Geometry: final body of the model. Coordinates: model frame, mm. A direction names the side the tool comes from. Coordinates: 2 decimals unless noted, no trailing zeros. Order: outer loops, then holes, each group sorted by start corner. A loop starts at its lowest first (then second) coordinate and runs counter-clockwise, first axis right, second up. Notation, with made-up numbers: (59.5, 3.5) -> (100.5, 3.5) arc R23 cw to (100.5, 25.5) -> close; hole circle Ø11 at (59, -11). An arc over 180 degrees is marked (long way). Answer in a Markdown table with one row per item. Add a question column.
1) Section query C-C on y = -177.8. Return the cut outline in (x, z) (3 decimals), then the cut area to 3 significant figures.
2) Pull-direction query (Y, two-part tool) for faces 3 (the face through (6, 196.85, -1)), 4 (the face through (9.21, -6.64, 124.28)), 5 (the face through (3.131, -46.94, 92.247)); classes: +Y half, -Y half, draft (parallel to the pull), parting line (faces both ways), or undercut.
3) Section query B-B on x = 38. Return the cut outline in (y, z).
4) Section query A-A on z = 44.45. Return the cut outline in (x, y).
5) Section query D-D on y = -93. Return the cut outline in (x, z) (3 decimals), then the cut area to 3 significant figures.
6) Ray query, line 1 (Y direction, x = 4, z = 44); line 2 (Y direction, x = 2.25, z = -44.45); line 3 (Z direction, x = 37.5, y = 130). Return the intervals inside material, ascending. Write a range as from..to.
7) Contact query for a flat-ended pin moving along its axis: P1, Ø1, axis at y = 13.5, z = 49.5, coming from the +X side. Output: stop coordinate, or through.
8) Set-up query: faces 1 (the face through (3.131, -43.793, 52.445)), 2 (the face through (30, -7, 127)). Return all of +Z, -Z, +X, -X, +Y, -Y with unobstructed straight access to the full face (end or side cutting, diameter ignored); none if empty.
```python
from build123d import *

# Parameters (mm, degrees)
BASE_EXTRUDE_THIN_DEPTH      = 196.85
BASE_EXTRUDE_THIN_DEPTH_BACK = 215.9
SKETCH3_R                    = 8.382
HOLES_DEPTH                  = 258.625377244


with BuildPart() as part:
    # Sketch1 → Base-Extrude-Thin (new, two sides)
    with BuildSketch(Plane(origin=(0, 0, 0), x_dir=(1, 0, 0), z_dir=(0, 1, 0))) as base_extrude_thin_sk:
        with BuildLine():
            Line((44.45, 133.35), (15.875, 133.35))
            ThreePointArc((15.875, 133.35), (4.649679849, 128.700320151), (0, 117.475))
            Line((0, 117.475), (0, 0))
            Line((0, 0), (0, -117.475))
            ThreePointArc((0, -117.475), (4.649679849, -128.700320151), (15.875, -133.35))
            Line((15.875, -133.35), (44.45, -133.35))
            Line((44.45, -133.35), (44.45, -127))
            Line((44.45, -127), (15.875, -127))
            ThreePointArc((15.875, -127), (9.139807909, -124.210192091), (6.35, -117.475))
            Line((6.35, -117.475), (6.35, 0))
            Line((6.35, 0), (6.35, 117.475))
            ThreePointArc((6.35, 117.475), (9.139807909, 124.210192091), (15.875, 127))
            Line((15.875, 127), (44.45, 127))
            Line((44.45, 127), (44.45, 133.35))
        make_face()
    extrude(amount=BASE_EXTRUDE_THIN_DEPTH)
    extrude(base_extrude_thin_sk.sketch, amount=-BASE_EXTRUDE_THIN_DEPTH_BACK)

    # Sketch3 (on Right Plane) → holes (cut, through all)
    with BuildSketch(Plane(origin=(0, 0, 0), x_dir=(0, 0, -1), z_dir=(1, 0, 0))):
        with Locations(Location((44.45, 168.275, 0), (0, 0, 180))):
            Circle(SKETCH3_R)
        with Locations(Location((44.45, 41.275, 0), (0, 0, 180))):
            Circle(SKETCH3_R)
        with Locations(Location((44.45, -41.275, 0), (0, 0, 180))):
            Circle(SKETCH3_R)
        with Locations(Location((44.45, -177.8, 0), (0, 0, 180))):
            Circle(SKETCH3_R)
        with Locations(Location((-44.45, -177.8, 0), (0, 0, 180))):
            Circle(SKETCH3_R)
        with Locations(Location((-98.425, -177.8, 0), (0, 0, 180))):
            Circle(SKETCH3_R)
        with Locations(Location((-98.425, -41.275, 0), (0, 0, 180))):
            Circle(SKETCH3_R)
        with Locations(Location((-44.45, -41.275, 0), (0, 0, 180))):
            Circle(SKETCH3_R)
        with Locations(Location((-44.45, 41.275, 0), (0, 0, 180))):
            Circle(SKETCH3_R)
        with Locations(Location((-98.425, 41.275, 0), (0, 0, 180))):
            Circle(SKETCH3_R)
        with Locations(Location((-98.425, 168.275, 0), (0, 0, 180))):
            Circle(SKETCH3_R)
        with Locations(Location((-44.45, 168.275, 0), (0, 0, 180))):
            Circle(SKETCH3_R)
        with Locations(Location((98.425, -177.8, 0), (0, 0, 180))):
            Circle(SKETCH3_R)
        with Locations(Location((98.425, -41.275, 0), (0, 0, 180))):
            Circle(SKETCH3_R)
        with Locations(Location((98.425, 41.275, 0), (0, 0, 180))):
            Circle(SKETCH3_R)
        with Locations(Location((98.425, 168.275, 0), (0, 0, 180))):
            Circle(SKETCH3_R)
    extrude(amount=HOLES_DEPTH, mode=Mode.SUBTRACT)


solid = part.part
```
Result:
| question | item | result |
|---|---|---|
| 1 | outline | (0, -117.475) arc R15.875 ccw to (15.875, -133.35) -> (44.45, -133.35) -> (44.45, -127) -> (15.875, -127) arc R9.525 cw to (6.35, -117.475) -> (6.35, -106.807) -> (0, -106.807) -> close; (0, -90.043) -> (6.35, -90.043) -> (6.35, -52.832) -> (0, -52.832) -> close; (0, -36.068) -> (6.35, -36.068) -> (6.35, 36.068) -> (0, 36.068) -> close; (0, 52.832) -> (6.35, 52.832) -> (6.35, 90.043) -> (0, 90.043) -> close; (0, 106.807) -> (6.35, 106.807) -> (6.35, 117.475) arc R9.525 cw to (15.875, 127) -> (44.45, 127) -> (44.45, 133.35) -> (15.875, 133.35) arc R15.875 ccw to (0, 117.475) -> close |
| 1 | area | 1,680 mm2 |
| 2 | face 3 | +Y half |
| 2 | face 4 | draft |
| 2 | face 5 | undercut |
| 3 | outline | (-215.9, -133.35) -> (196.85, -133.35) -> (196.85, -127) -> (-215.9, -127) -> close; (-215.9, 127) -> (196.85, 127) -> (196.85, 133.35) -> (-215.9, 133.35) -> close |
| 4 | outline | (0, -215.9) -> (6.35, -215.9) -> (6.35, -186.18) -> (0, -186.18) -> close; (0, -169.42) -> (6.35, -169.42) -> (6.35, -49.66) -> (0, -49.66) -> close; (0, -32.89) -> (6.35, -32.89) -> (6.35, 32.89) -> (0, 32.89) -> close; (0, 49.66) -> (6.35, 49.66) -> (6.35, 159.89) -> (0, 159.89) -> close; (0, 176.66) -> (6.35, 176.66) -> (6.35, 196.85) -> (0, 196.85) -> close |
| 5 | outline | (0, -117.475) arc R15.875 ccw to (15.875, -133.35) -> (44.45, -133.35) -> (44.45, -127) -> (15.875, -127) arc R9.525 cw to (6.35, -117.475) -> (6.35, 117.475) arc R9.525 cw to (15.875, 127) -> (44.45, 127) -> (44.45, 133.35) -> (15.875, 133.35) arc R15.875 ccw to (0, 117.475) -> close |
| 5 | area | 2,110 mm2 |
| 6 | line 1 | -215.9..-186.17, -169.43..-49.64, -32.91..32.91, 49.64..159.91, 176.64..196.85 |
| 6 | line 2 | -215.9..-186.18, -169.42..-49.66, -32.89..32.89, 49.66..159.89, 176.66..196.85 |
| 6 | line 3 | -133.35..-127, 127..133.35 |
| 7 | P1 | x = 6.35 |
| 8 | face 1 | +X, -X |
| 8 | face 2 | +X, +Y, -Y |
